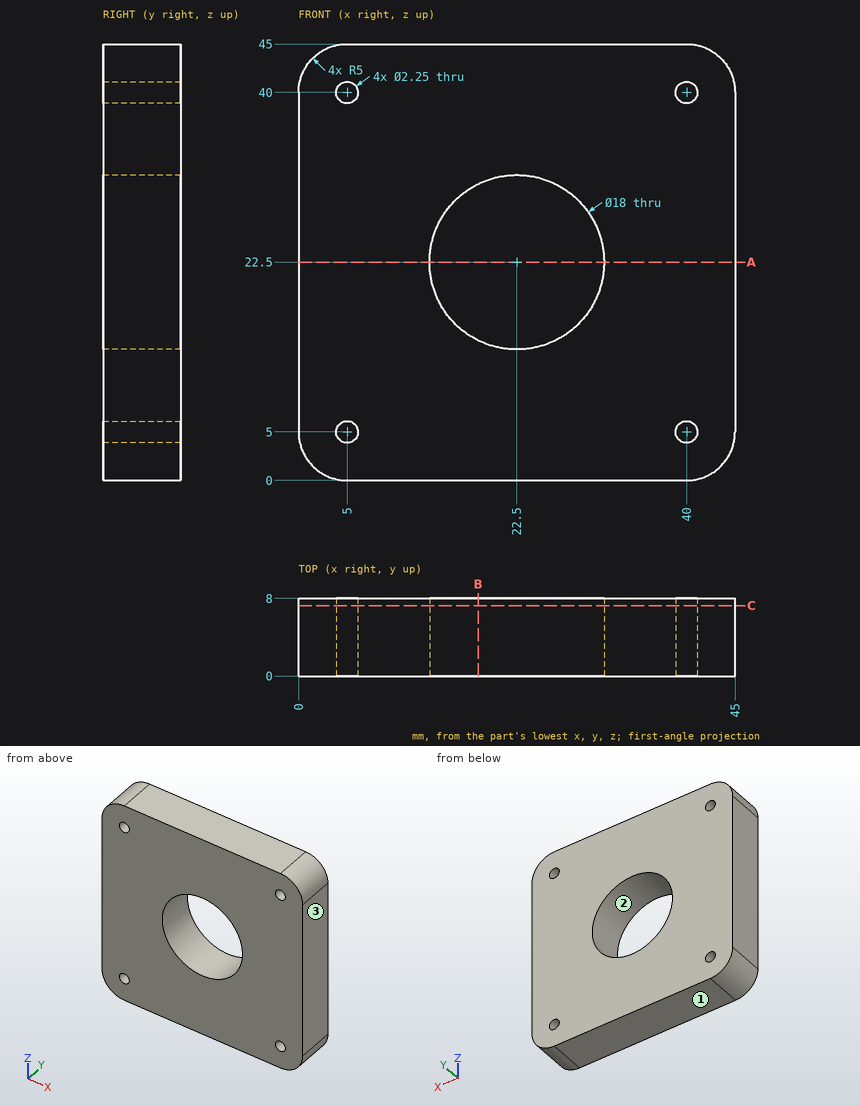
Could you check a few things on this drawing? It's one solid part, dimensions in mm from its lowest x, y, z. Give positions to 0.01 mm unless a question says otherwise; leave off trailing zeros. Write each loop counter-clockwise with the first axis right and the second up, starting at its lowest first coordinate (ties: lowest second). Pieces come first, ordered by that corner, then holes. Notation, with made-up numbers: M -25,65.25 L -18,65.25 A20 ccw -18,83.25 Z; hole C -11.5,-3.5 d2. An arc over 180 degrees is marked long. Put each result on its own line as item: value. Start each with the question number.
Item 1: Thinking about a two-plate mould opening in Z: for the marked faces 1, 2 and 3, which applies, +Z half, -Z half, draft (parallel to the pull), parting line (faces both ways), or undercut?
Item 2: If we section it at B-B, the plane x = 18.5: Write out the boundary of the cut face in (y, z), then the cut area to 3 significant figures.
Item 3: If we section it at A-A, the plane z = 22.5: Write out the boundary of the cut face in (x, y).
Item 4: I need wall thicknesses on L1, parallel to X at y = 5.75, z = 40 (3 decimals); L2, parallel to X at y = 5, z = 24; L3, parallel to X at y = 1, z = 20. Which ranges of each line are inside material? Lowest first, please. Write a range as from..to.
Item 5: If we section it at C-C, the plane y = 7.25: Write out the boundary of the cut face in (x, z) (3 decimals), then the cut area to 3 significant figures.
Values:
1. face 1: -Z half
1. face 2: undercut
1. face 3: draft
2. outline: M 0,0 L 8,0 L 8,14.44 L 0,14.44 Z; M 0,30.56 L 8,30.56 L 8,45 L 0,45 Z
2. area: 231 mm²
3. outline: M 0,0 L 13.5,0 L 13.5,8 L 0,8 Z; M 31.5,0 L 45,0 L 45,8 L 31.5,8 Z
4. L1: 0..3.875, 6.125..38.875, 41.125..45
4. L2: 0..13.63, 31.37..45
4. L3: 0..13.85, 31.15..45
5. outline: M 0,5 A5 ccw 5,0 L 40,0 A5 ccw 45,5 L 45,40 A5 ccw 40,45 L 5,45 A5 ccw 0,40 Z; hole C 5,5 d2.25; hole C 5,40 d2.25; hole C 22.5,22.5 d18; hole C 40,5 d2.25; hole C 40,40 d2.25
5. area: 1,730 mm²
